```python
from build123d import *

# Parameters (mm, degrees)
CYLINDER001_R     = 1.8
CYLINDER001_DEPTH = 10
BOX002_W          = 18
BOX002_H          = 6
BOX002_DEPTH      = 7
FILLET_R          = 1
CYLINDER_R        = 3
CYLINDER_DEPTH    = 3
BOX_W             = 30
BOX_H             = 6
BOX_DEPTH         = 3
BOX001_W          = 22
BOX001_H          = 6
BOX001_DEPTH      = 9
FILLET001_R       = 1


with BuildPart() as bolt_hole:
    # Cylinder001 → Cylinder001 (new body)
    with BuildSketch(Plane(origin=(-15, 0, 0), x_dir=(1, 0, 0), z_dir=(0, 0, 1))):
        Circle(CYLINDER001_R)
    extrude(amount=CYLINDER001_DEPTH)


with BuildPart() as central_hole_fillet:
    # Box002 → Box002 (new body)
    with BuildSketch(Plane(origin=(-9, -3, 3), x_dir=(1, 0, 0), z_dir=(0, 0, 1))):
        with Locations((9, 3)):
            Rectangle(BOX002_W, BOX002_H)
    extrude(amount=BOX002_DEPTH)

    # Fillet
    fillet_edges = [central_hole_fillet.edges().sort_by_distance(p)[0] for p in [
        (-9, 0, 10),
        (-9, 0, 3),
        (9, 0, 10),
        (9, 0, 3),
    ]]
    fillet(fillet_edges, radius=FILLET_R)


with BuildPart() as extract_fusion:
    # Part__Mirroring001: instance of bolt hole
    add(bolt_hole.part.mirror(Plane(origin=(0, 0, 0), x_dir=(0, -1, 0), z_dir=(1, 0, 0))))

    # Fusion001: union bolt hole, central hole fillet
    add(bolt_hole.part)
    add(central_hole_fillet.part)


with BuildPart() as end_cylinder:
    # Cylinder → Cylinder (new body)
    with BuildSketch(Plane(origin=(-15, 0, 0), x_dir=(1, 0, 0), z_dir=(0, 0, 1))):
        Circle(CYLINDER_R)
    extrude(amount=CYLINDER_DEPTH)


with BuildPart() as part_mirroring:
    # Part__Mirroring: instance of end cylinder
    add(end_cylinder.part.mirror(Plane(origin=(0, 0, 0), x_dir=(0, -1, 0), z_dir=(1, 0, 0))))


with BuildPart() as bottom_cube:
    # Box → Box (new body)
    with BuildSketch(Plane(origin=(-15, -3, 0), x_dir=(1, 0, 0), z_dir=(0, 0, 1))):
        with Locations((15, 3)):
            Rectangle(BOX_W, BOX_H)
    extrude(amount=BOX_DEPTH)


with BuildPart() as top_cube_fillet:
    # Box001 → Box001 (new body)
    with BuildSketch(Plane(origin=(-11, -3, 3), x_dir=(1, 0, 0), z_dir=(0, 0, 1))):
        with Locations((11, 3)):
            Rectangle(BOX001_W, BOX001_H)
    extrude(amount=BOX001_DEPTH)

    # Fillet001
    fillet001_edges = [top_cube_fillet.edges().sort_by_distance(p)[0] for p in [
        (-11, 0, 12),
        (11, 0, 12),
    ]]
    fillet(fillet001_edges, radius=FILLET001_R)


with BuildPart() as wire_holder:
    # Fusion base: copy of end cylinder
    add(end_cylinder.part)

    # Fusion: union Part__Mirroring, bottom cube, top cube fillet
    add(part_mirroring.part)
    add(bottom_cube.part)
    add(top_cube_fillet.part)

    # Cut: cut extract fusion
    add(extract_fusion.part, mode=Mode.SUBTRACT)


solid = wire_holder.part
```
Model file for the job. Use its own axes, mm. A direction names the side the tool comes from. Give positions to 0.01 mm unless a question says otherwise; leave off trailing zeros. Loops run counter-clockwise (first coordinate to the right, second up) from the corner with the lowest first, then second, coordinate; pieces in that order, holes last. Notation, with made-up numbers: (-11, 77) - (30, 77) arc R16 cw to (30, 83) - close; hole circle Ø2 at (-31.5, 9). An arc over 180 degrees is marked (long way). One line per item, written item: value. Start each with the question number.
1. Slice it at B-B (x = 2). List the corners of the cut face in (y, z).
2. Pull direction Z, two halves, no side cores. Call faces 6 (the cylindrical face through (-8.715, 0.042, 9.699)), 7 (the flat face through (0, 0, 0)), 8 (the cylindrical face through (-13.283, 0.541, 1.479)), 9 (the flat face through (-13, 0, 3)): pulls with the +Z half, pulls with the -Z half, needs draft (parallel to the pull), parting line crosses it, or undercut.
3. Pin check, flat tips, straight feed: pin 1 (2 mm diameter, centred on x = 0, y = 2, fed in from -Z); pin 2 (2 mm diameter, centred on y = -2, z = 7.5, fed in from +X); pin 3 (1.5 mm diameter, centred on y = 0.5, z = 6, fed in from -X). Stop position of each tip, or through.
4. Slice it at A-A (y = 0). List the corners of the cut face in (x, z).
5. Probe L1, parallel to X at y = -1.15, z = 4; L2, parallel to Z at x = -6, y = -2.5; L3, parallel to Y at x = -15, z = 2.2. List the from-to ranges inside material, lowest first. Write a range as from..to.
6. Slice it at D-D (z = 10.5). List the corners of the cut face in (x, y).
7. Slice it at C-C (z = 6.5). List the corners of the cut face in (x, y).
8. Which spindle directions (+Z, -Z, +X, -X, +Y, -Y) get a long thin tool onto all of the face, cutting with end or side? Do faces 1 (the cylindrical face through (-18, 0, 1)), 2 (the flat face through (11, 0, 7)), 3 (the flat face through (-11, 0, 7)), 4 (the cylindrical face through (13.283, 0.541, 1.479)), 5 (the flat face through (0, 0, 3)). Say none if no direction does.
Solution:
1. outline: (-3, 0) - (3, 0) - (3, 3) - (-3, 3) - close; (-3, 10) - (3, 10) - (3, 12) - (-3, 12) - close
2. face 6: undercut
2. face 7: pulls with the -Z half
2. face 8: needs draft
2. face 9: pulls with the +Z half
3. pin 1: stops at z = 0
3. pin 2: stops at x = 11
3. pin 3: stops at x = -11
4. outline: (-18, 0) - (-16.8, 0) - (-16.8, 3) - (-18, 3) - close; (-13.2, 0) - (13.2, 0) - (13.2, 3) - (11, 3) - (11, 11) arc R1 ccw to (10, 12) - (-10, 12) arc R1 ccw to (-11, 11) - (-11, 3) - (-13.2, 3) - close; (16.8, 0) - (18, 0) - (18, 3) - (16.8, 3) - close; hole (-9, 4) arc R1 ccw to (-8, 3) - (8, 3) arc R1 ccw to (9, 4) - (9, 9) arc R1 ccw to (8, 10) - (-8, 10) arc R1 ccw to (-9, 9) - close
5. L1: x = -11..-9, 9..11
5. L2: z = 0..3, 10..12
5. L3: y = -3..-1.8, 1.8..3
6. outline: (-11, -3) - (11, -3) - (11, 3) - (-11, 3) - close
7. outline: (-11, -3) - (-9, -3) - (-9, 3) - (-11, 3) - close; (9, -3) - (11, -3) - (11, 3) - (9, 3) - close
8. face 1: +Z, -Z, -X
8. face 2: +Z, +X, +Y, -Y
8. face 3: +Z, -X, +Y, -Y
8. face 4: +Z, -Z
8. face 5: +Y, -Y
